Design review of the part built by this model. Coordinates are the model's own, in mm. A direction names the side the tool comes from. Round coordinates to 2 decimals unless told otherwise and drop trailing zeros. Loops run counter-clockwise (first coordinate to the right, second up) from the corner with the lowest first, then second, coordinate; pieces in that order, holes last. Notation, with made-up numbers: (18, 2) -> (27, 2) arc R21 ccw to (27, 18) -> close; hole circle Ø9 at (12, -39). An arc over 180 degrees is marked (long way). Answer as CSV lines item,"result". Start each with the question number.
(1) To check wall thickness, follow line 1 (Y direction, x = 58.5, z = 5.75); line 2 (Z direction, x = 48, y = 0) (3 decimals); line 3 (Y direction, x = 155.5, z = 5.5). State the ranges of each line that lie inside material, in increasing order. Write a range as from..to.
(2) Draft analysis for pull direction Z (two halves, no side actions). For faces 1 (the face through (311.15, -3, 0)), 2 (the face through (153, 8, -12.596)), 3 (the face through (153.397, -6.142, -8.589)), state which applies: +Z half, -Z half, draft (parallel to the pull), parting line (faces both ways), or undercut.
(3) For P1, Ø1.7, axis at x = 60, z = 0, coming from the +Y side; P2, Ø4.5, axis at x = 56, y = -0.5, coming from the -Z side; P3, Ø1.7, axis at x = 85.5, y = -1.5, coming from the +Z side, all flat-tipped, find the tip position at first contact; note any pin that passes through.
(4) Take a section at A-A, the plane z = 0. Write out the cut boundary in (x, y) (3 decimals), and give its area (3 significant figures).
(5) Take a section at B-B, the plane y = 0. Write out the cut boundary in (x, z) (3 decimals), and give its area (3 significant figures).
(6) Machinability: for faces 4 (the face through (75, 5, 0)), 5 (the face through (235, 0, 5)), 6 (the face through (75, -5, 0)), which of the approach directions +Z, -Z, +X, -X, +Y, -Y give a long, thin tool a straight path to every point of the face, cutting with its end or side? Answer none if there is none.
from build123d import *

# Parameters (mm, degrees)
SKETCH1_W           = 10
SKETCH1_H           = 10
SKETCH1_R           = 2.605
BOSS_EXTRUDE1_DEPTH = 311.15
CIRPATTERN1_COUNT   = 4
SKETCH2_R           = 6.35
CUT_EXTRUDE1_DEPTH  = 30


with BuildPart() as part:
    # Sketch1 → Boss-Extrude1 (new body)
    with BuildSketch(Plane(origin=(0, 0, 0), x_dir=(0, 0, -1), z_dir=(1, 0, 0))):
        Rectangle(SKETCH1_W, SKETCH1_H)
        Circle(SKETCH1_R, mode=Mode.SUBTRACT)
        Polygon((7.474873734, 9.921463197), (2.553410537, 5), (5, 5), (5, 3.203948776), (9.596194078, 7.800142853), align=None)
        Polygon((9.596194078, 3.24), (12.596194078, 3.24), (12.596194078, 12.596194078), (3.24, 12.596194078), (3.24, 9.921463197), (7.474873734, 9.921463197), (9.596194078, 7.800142853), align=None)
    boss_extrude1 = extrude(amount=BOSS_EXTRUDE1_DEPTH)

    # CirPattern1: Boss-Extrude1 ×4 about axis
    cirpattern1_axis = Axis((0, 0, 0), (1, 0, 0))
    for i in range(1, CIRPATTERN1_COUNT):
        add(boss_extrude1.rotate(cirpattern1_axis, i * 360 / CIRPATTERN1_COUNT))

    # Sketch2 → Cut-Extrude1 (cut)
    with BuildSketch(Plane.XY.offset(12.596194078)):
        with Locations((155.575, 0)):
            Circle(SKETCH2_R)
    extrude(amount=-CUT_EXTRUDE1_DEPTH, mode=Mode.SUBTRACT)


solid = part.part
The answers:
1,line 1,"-12.6..-9.92, -8.2..-3.95, 3.3..7.55, 9.6..12.6"
1,line 2,"-5..-2.605, 2.605..5"
1,line 3,"-12.6..-9.92, -7.95..-6.35, 6.35..7.3, 9.6..12.6"
2,face 1,"draft"
2,face 2,"-Z half"
2,face 3,"undercut"
3,P1,"y = 5"
3,P2,"z = -5.2"
3,P3,"z = 5"
4,outline,"(0, -5) -> (151.661, -5) arc R6.35 cw to (149.784, -2.605) -> (0, -2.605) -> close; (0, 2.605) -> (149.784, 2.605) arc R6.35 cw to (151.661, 5) -> (0, 5) -> close; (159.489, -5) -> (311.15, -5) -> (311.15, -2.605) -> (161.366, -2.605) arc R6.35 cw to start; (159.489, 5) arc R6.35 cw to (161.366, 2.605) -> (311.15, 2.605) -> (311.15, 5) -> close"
4,area,"1,440 mm²"
5,outline,"(0, -5) -> (149.225, -5) -> (149.225, -2.605) -> (0, -2.605) -> close; (0, 2.605) -> (149.225, 2.605) -> (149.225, 5) -> (0, 5) -> close; (161.925, -5) -> (311.15, -5) -> (311.15, -2.605) -> (161.925, -2.605) -> close; (161.925, 2.605) -> (311.15, 2.605) -> (311.15, 5) -> (161.925, 5) -> close"
5,area,"1,430 mm²"
6,face 4,"+X, -X, +Y"
6,face 5,"+Z, +X, -X"
6,face 6,"+X, -X, -Y"
